The listing builds one solid part. Answer for the finished solid, in the listing's coordinates (mm). Face numbers are marked on the shaded views. A direction names the side the tool comes from. Round coordinates to 2 decimals unless told otherwise and drop trailing zeros. Write each loop counter-clockwise with the first axis right and the second up, starting at its lowest first coordinate (ties: lowest second). Pieces come first, ordered by that corner, then holes. Notation, with made-up numbers: (-33.75, 0) - (5.25, 0) arc R18 cw to (5.25, 24) - close; hole circle Ø7 at (60, -14.5). An arc over 180 degrees is marked (long way). Answer as CSV lines item,"result". Start each with the question number.
Item 1: Flat-ended cylindrical pins translate along their axes: pin 1 (3 mm diameter, centred on y = 0.5, z = 13, fed in from +X); pin 2 (1.5 mm diameter, centred on y = 1.5, z = 12, fed in from -X); pin 3 (2 mm diameter, centred on x = 0, z = 24.5, fed in from +Y). Find the tip coordinate at first contact, or state that the pin passes through.
Item 2: Which of the six approach directions +Z, -Z, +X, -X, +Y, -Y give full straight-line access (tool end or side, diameter ignored) to the marked faces 1 and 2?
Item 3: Straight lines are drawn through the part: line 1 along Y through (x, z) = (0, 4.75); line 2 along Z through (x, y) = (1.75, -2); line 3 along X through (y, z) = (-1.75, 2.5). For each, find the intervals that lie inside material, in ascending order. Write a range as [from, to].
Item 4: A cutting plane is placed at C-C on z = 18.5. Determine the outline of the cut face in (x, y).
Item 5: A cutting plane is placed at B-B on y = 0. Determine the outline of the cut face in (x, z).
```python
from build123d import *

# Parameters (mm, degrees)
BOSS_EXTRUDE1_DEPTH = 3.5
SKETCH2_OUTSIDE_W   = 31.08
SKETCH2_OUTSIDE_H   = 30.448
SKETCH2_OUTSIDE_R   = 4
CUT_EXTRUDE1_DEPTH  = 5
CUT_EXTRUDE1_DRAFT  = -60
SKETCH3_R           = 2.5
BOSS_EXTRUDE2_DEPTH = 25


with BuildPart() as part:
    # Sketch1 → Boss-Extrude1 (new body)
    with BuildSketch(Plane.XY):
        Polygon((1.77607371, 4.2636716), (-2.804411064, 3.669960751), (-4.580484774, -0.593710848), (-1.77607371, -4.2636716), (2.804411064, -3.669960751), (4.580484774, 0.593710848), align=None)
    extrude(amount=BOSS_EXTRUDE1_DEPTH)


with BuildPart() as cut_extrude1_tool:
    # Sketch2 outside → Cut-Extrude1 (with draft: the straight prism first)
    with BuildSketch(Plane(origin=(0, 0, 0), x_dir=(-1, 0, 0), z_dir=(0, 0, -1))):
        Rectangle(SKETCH2_OUTSIDE_W, SKETCH2_OUTSIDE_H)
        Circle(SKETCH2_OUTSIDE_R, mode=Mode.SUBTRACT)
    extrude(amount=-CUT_EXTRUDE1_DEPTH)
    # Cut-Extrude1: the draft: its side faces are tilted about the plane it starts from
    cut_extrude1_sides = [cut_extrude1_tool.faces().sort_by_distance(p)[0] for p in [
        (0, -15.224, 2.5),
        (-15.54, 0, 2.5),
        (0, 15.224, 2.5),
        (15.54, 0, 2.5),
        (4, 0, 2.5),
    ]]
    draft(cut_extrude1_sides, Plane(origin=(0, 0, 0), x_dir=(-1, 0, 0), z_dir=(0, 0, -1)), CUT_EXTRUDE1_DRAFT)


with BuildPart() as part_1:
    add(part.part)

    # Cut-Extrude1: cut by cut_extrude1_tool
    add(cut_extrude1_tool.part, mode=Mode.SUBTRACT)

    # Sketch3 → Boss-Extrude2 (add)
    with BuildSketch(Plane.XY.offset(3.5)):
        Circle(SKETCH3_R)
    extrude(amount=BOSS_EXTRUDE2_DEPTH)


solid = part_1.part
```
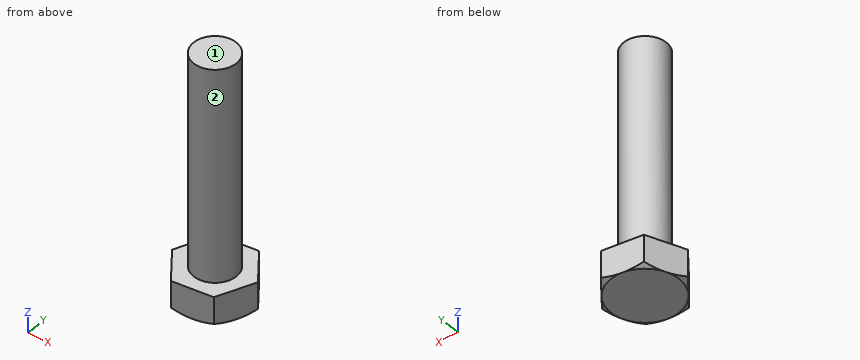
Geometry says:
1,pin 1,"stops at x = 2.5"
1,pin 2,"stops at x = -2.38"
1,pin 3,"stops at y = 2.5"
2,face 1,"+Z, +X, -X, +Y, -Y"
2,face 2,"+Z"
3,line 1,"y = [-2.5, 2.5]"
3,line 2,"z = [0, 3.5]"
3,line 3,"x = [-3.7, 3.6]"
4,outline,"circle Ø5 at (0, 0)"
5,outline,"(-4.33, 0.19) - (-4, 0) - (4, 0) - (4.33, 0.19) - (4.33, 3.5) - (2.5, 3.5) - (2.5, 28.5) - (-2.5, 28.5) - (-2.5, 3.5) - (-4.33, 3.5) - close"
